from build123d import *

# Parameters (mm, degrees)
F1_DEPTH = 18
F2_T     = -0.7
F4_W     = 0.7
F4_H     = 118.6
F5_DEPTH = 2


with BuildPart() as f1:
    # F0 (on Top) → F1 (new body)
    with BuildSketch(Plane.XY):
        Polygon((37.585583, 77.584211), (-2.414417, 77.584211), (-2.414417, -42.415789), (7.585583, -42.415789), align=None)
    extrude(amount=F1_DEPTH)

    # F2
    f2_openings = [f1.faces().sort_by_distance(p)[0] for p in [
        (11.585583, 29.584211, 18),
    ]]
    offset(amount=F2_T, openings=f2_openings)

    # F4 (on face) → F5 (join)
    with BuildSketch(Plane.XY.offset(0.7)):
        with Locations((1.135583, 17.584211)):
            Rectangle(F4_W, F4_H)
    extrude(amount=F5_DEPTH)


solid = f1.part
Check sheet for the modelled part. Datum: model origin and axes. Units: mm. A direction names the side the tool comes from. Coordinates: 2 decimals unless noted, no trailing zeros. Write each loop counter-clockwise with the first axis right and the second up, starting at its lowest first coordinate (ties: lowest second). Pieces come first, ordered by that corner, then holes.
Item 1: Cross-section at A-A on z = 12. Record the boundary of the cut face in (x, y).
Numbers:
outline: (-2.41, -42.42) - (7.59, -42.42) - (37.59, 77.58) - (-2.41, 77.58) - close; hole (-1.71, -41.72) - (7.04, -41.72) - (36.69, 76.88) - (-1.71, 76.88) - close
Item 2: Cross-section at C-C on y = 32.5. Record the boundary of the cut face in (x, z).
Numbers:
outline: (-2.41, 0) - (26.31, 0) - (26.31, 18) - (25.59, 18) - (25.59, 0.7) - (1.49, 0.7) - (1.49, 2.7) - (0.79, 2.7) - (0.79, 0.7) - (-1.71, 0.7) - (-1.71, 18) - (-2.41, 18) - close
Item 3: Mould release check, pull along Y, two halves, no side actions. Record for faces 3 (the face through (18, 77.584, 9)), 4 (the face through (-2, 18, 18)), 5 (the face through (-1.714, 18, 9)), 6 (the face through (21.656, 16.754, 9.229)): released by +Y, released by -Y, zero draft, split by the parting line, or undercut.
Numbers:
face 3: released by +Y
face 4: zero draft
face 5: undercut
face 6: undercut
Item 4: Access from +Z, -Z, +X, -X, +Y, -Y to the whole of each face (thin tool, end or side, straight path). Record for faces 1 (the face through (13, 32, 0)), 2 (the face through (3, -41.716, 9)).
Numbers:
face 1: -Z, +X, -X, +Y, -Y
face 2: +Z
Item 5: Cross-section at D-D on y = 18. Record the boundary of the cut face in (x, z).
Numbers:
outline: (-2.41, 0) - (22.69, 0) - (22.69, 18) - (21.97, 18) - (21.97, 0.7) - (1.49, 0.7) - (1.49, 2.7) - (0.79, 2.7) - (0.79, 0.7) - (-1.71, 0.7) - (-1.71, 18) - (-2.41, 18) - close
Item 6: Depth check by flat-ended pin: pin 1 Ø6 at (y, z) = (30.5, 14.5) entering from +X; pin 2 Ø8 at (y, z) = (57, 9) entering from +X; pin 3 Ø4 at (y, z) = (7.5, 12) entering from +X. Enter the tip coordinate at first touch or a pass-through.
Numbers:
pin 1: stops at x = 26.56
pin 2: stops at x = 33.44
pin 3: stops at x = 20.56
Item 7: Cross-section at B-B on x = 4. Record the boundary of the cut face in (y, z), then the cut area to 3 significant figures.
Numbers:
outline: (-42.42, 0) - (77.58, 0) - (77.58, 18) - (76.88, 18) - (76.88, 0.7) - (-41.72, 0.7) - (-41.72, 18) - (-42.42, 18) - close
area: 108 mm2
Item 8: Scan lines: probe 1 along X at (y, z) = (1, 1); probe 2 along X at (y, z) = (20, 1); probe 3 along Y at (x, z) = (2.5, 9.25). Record each from-to range of solid material in increasing order.
Numbers:
probe 1: x = -2.41 to -1.71, 0.79 to 1.49, 17.72 to 18.44
probe 2: x = -2.41 to -1.71, 0.79 to 1.49, 22.47 to 23.19
probe 3: y = -42.42 to -41.72, 76.88 to 77.58
